```python
from build123d import *

# Parameters (mm, degrees)
F0_R     = 41.5925
F0_R_2   = 8.89
F1_DEPTH = 6.35
F2_R     = 41.5925
F2_R_2   = 33.9725
F3_DEPTH = 3.175
F4_R     = 41.5925
F4_R_2   = 33.9725
F4_R_3   = 0.762
F5_DEPTH = 2.54
F7_DEPTH = 6.985
F8_R     = 41.5925
F8_W     = 50.8
F8_H     = 50.8
F8_R_2   = 8.89
F8_R_3   = 8.382
F9_DEPTH = 12.7


with BuildPart() as f1:
    # F0 (on Top) → F1 (new body)
    with BuildSketch(Plane.XY):
        Circle(F0_R)
        Circle(F0_R_2, mode=Mode.SUBTRACT)
    extrude(amount=F1_DEPTH)

    # F2 (on face) → F3 (join)
    with BuildSketch(Plane.XY.offset(6.35)):
        Circle(F2_R)
        Circle(F2_R_2, mode=Mode.SUBTRACT)
    extrude(amount=F3_DEPTH)

    # F4 (on face) → F5 (join)
    with BuildSketch(Plane.XY.offset(9.525)):
        Circle(F4_R)
        Circle(F4_R_2, mode=Mode.SUBTRACT)
        Circle(F4_R_2)
        with Locations((-18.7126454725, -21.5955440872)):
            Circle(F4_R_3, mode=Mode.SUBTRACT)
        with Locations((-14.2875, -24.7466759131)):
            Circle(F4_R_3, mode=Mode.SUBTRACT)
        with Locations((-9.3459670518, -27.0033983948)):
            Circle(F4_R_3, mode=Mode.SUBTRACT)
        with Locations((-4.0666465037, -28.2841477017)):
            Circle(F4_R_3, mode=Mode.SUBTRACT)
        with Locations((-6.5563218998, -21.8996402515)):
            Circle(F4_R_3, mode=Mode.SUBTRACT)
        with Locations((-1.3291907889, -22.8213244981)):
            Circle(F4_R_3, mode=Mode.SUBTRACT)
        with Locations((-22.4614671823, -17.6638930313)):
            Circle(F4_R_3, mode=Mode.SUBTRACT)
        with Locations((-25.3984729453, -13.0938228584)):
            Circle(F4_R_3, mode=Mode.SUBTRACT)
        with Locations((-27.417511721, -8.0505078117)):
            Circle(F4_R_3, mode=Mode.SUBTRACT)
        with Locations((-21.4813733112, -7.8185804764)):
            Circle(F4_R_3, mode=Mode.SUBTRACT)
        with Locations((-28.4456101875, -2.7162264374)):
            Circle(F4_R_3, mode=Mode.SUBTRACT)
        with Locations((-22.705428858, -2.6538840169)):
            Circle(F4_R_3, mode=Mode.SUBTRACT)
        with Locations((-15.6874838417, -16.6277614464)):
            Circle(F4_R_3, mode=Mode.SUBTRACT)
        with Locations((-11.43, -19.7973407305)):
            Circle(F4_R_3, mode=Mode.SUBTRACT)
        with Locations((-19.0992513689, -12.5617752387)):
            Circle(F4_R_3, mode=Mode.SUBTRACT)
        with Locations((-5.2980963686, -16.3058639719)):
            Circle(F4_R_3, mode=Mode.SUBTRACT)
        with Locations((-10.0775781506, -13.8705963686)):
            Circle(F4_R_3, mode=Mode.SUBTRACT)
        with Locations((-4.0531338589, -10.6872356539)):
            Circle(F4_R_3, mode=Mode.SUBTRACT)
        with Locations((-16.3058639719, -5.2980963686)):
            Circle(F4_R_3, mode=Mode.SUBTRACT)
        with Locations((-13.8705963686, -10.0775781506)):
            Circle(F4_R_3, mode=Mode.SUBTRACT)
        with Locations((-11.0978649732, -2.7353780428)):
            Circle(F4_R_3, mode=Mode.SUBTRACT)
        with Locations((-8.5554778516, -7.5794919837)):
            Circle(F4_R_3, mode=Mode.SUBTRACT)
        with Locations((-2.8575, -4.9493351826)):
            Circle(F4_R_3, mode=Mode.SUBTRACT)
        with Locations((1.3596532447, -28.5426342172)):
            Circle(F4_R_3, mode=Mode.SUBTRACT)
        with Locations((6.7368115822, -27.7695155648)):
            Circle(F4_R_3, mode=Mode.SUBTRACT)
        with Locations((3.9695973415, -22.5127052339)):
            Circle(F4_R_3, mode=Mode.SUBTRACT)
        with Locations((9.0543834517, -20.9904202033)):
            Circle(F4_R_3, mode=Mode.SUBTRACT)
        with Locations((11.8704839965, -25.9927342673)):
            Circle(F4_R_3, mode=Mode.SUBTRACT)
        with Locations((16.575126191, -23.2765078298)):
            Circle(F4_R_3, mode=Mode.SUBTRACT)
        with Locations((0, -17.145)):
            Circle(F4_R_3, mode=Mode.SUBTRACT)
        with Locations((5.2980963686, -16.3058639719)):
            Circle(F4_R_3, mode=Mode.SUBTRACT)
        with Locations((1.3777342553, -11.3466624309)):
            Circle(F4_R_3, mode=Mode.SUBTRACT)
        with Locations((10.0775781506, -13.8705963686)):
            Circle(F4_R_3, mode=Mode.SUBTRACT)
        with Locations((13.6510454063, -18.3365361864)):
            Circle(F4_R_3, mode=Mode.SUBTRACT)
        with Locations((20.6807001389, -19.7190077531)):
            Circle(F4_R_3, mode=Mode.SUBTRACT)
        with Locations((17.5117759697, -14.6941247574)):
            Circle(F4_R_3, mode=Mode.SUBTRACT)
        with Locations((6.4929800551, -9.4067055872)):
            Circle(F4_R_3, mode=Mode.SUBTRACT)
        with Locations((10.1207623732, -5.3117858565)):
            Circle(F4_R_3, mode=Mode.SUBTRACT)
        with Locations((2.8575, -4.9493351826)):
            Circle(F4_R_3, mode=Mode.SUBTRACT)
        with Locations((13.8705963686, -10.0775781506)):
            Circle(F4_R_3, mode=Mode.SUBTRACT)
        with Locations((20.4284421578, -10.2595492594)):
            Circle(F4_R_3, mode=Mode.SUBTRACT)
        with Locations((16.3058639719, -5.2980963686)):
            Circle(F4_R_3, mode=Mode.SUBTRACT)
        with Locations((24.0388197007, -15.4488113588)):
            Circle(F4_R_3, mode=Mode.SUBTRACT)
        with Locations((26.5281136859, -10.6202546705)):
            Circle(F4_R_3, mode=Mode.SUBTRACT)
        with Locations((22.2438057415, -5.2718788052)):
            Circle(F4_R_3, mode=Mode.SUBTRACT)
        with Locations((28.0586125243, -5.4078543076)):
            Circle(F4_R_3, mode=Mode.SUBTRACT)
        with Locations((-28.4456101875, 2.7162264374)):
            Circle(F4_R_3, mode=Mode.SUBTRACT)
        with Locations((-22.705428858, 2.6538840169)):
            Circle(F4_R_3, mode=Mode.SUBTRACT)
        with Locations((-27.417511721, 8.0505078117)):
            Circle(F4_R_3, mode=Mode.SUBTRACT)
        with Locations((-21.4813733112, 7.8185804764)):
            Circle(F4_R_3, mode=Mode.SUBTRACT)
        with Locations((-25.3984729453, 13.0938228584)):
            Circle(F4_R_3, mode=Mode.SUBTRACT)
        with Locations((-22.4614671823, 17.6638930313)):
            Circle(F4_R_3, mode=Mode.SUBTRACT)
        with Locations((-17.145, 0)):
            Circle(F4_R_3, mode=Mode.SUBTRACT)
        with Locations((-11.0978649732, 2.7353780428)):
            Circle(F4_R_3, mode=Mode.SUBTRACT)
        with Locations((-16.3058639719, 5.2980963686)):
            Circle(F4_R_3, mode=Mode.SUBTRACT)
        with Locations((-13.8705963686, 10.0775781506)):
            Circle(F4_R_3, mode=Mode.SUBTRACT)
        with Locations((-5.715, 0)):
            Circle(F4_R_3, mode=Mode.SUBTRACT)
        with Locations((-2.8575, 4.9493351826)):
            Circle(F4_R_3, mode=Mode.SUBTRACT)
        with Locations((-8.5554778516, 7.5794919837)):
            Circle(F4_R_3, mode=Mode.SUBTRACT)
        with Locations((-19.0992513689, 12.5617752387)):
            Circle(F4_R_3, mode=Mode.SUBTRACT)
        with Locations((-15.6874838417, 16.6277614464)):
            Circle(F4_R_3, mode=Mode.SUBTRACT)
        with Locations((-11.43, 19.7973407305)):
            Circle(F4_R_3, mode=Mode.SUBTRACT)
        with Locations((-10.0775781506, 13.8705963686)):
            Circle(F4_R_3, mode=Mode.SUBTRACT)
        with Locations((-4.0531338589, 10.6872356539)):
            Circle(F4_R_3, mode=Mode.SUBTRACT)
        with Locations((-5.2980963686, 16.3058639719)):
            Circle(F4_R_3, mode=Mode.SUBTRACT)
        with Locations((-18.7126454725, 21.5955440872)):
            Circle(F4_R_3, mode=Mode.SUBTRACT)
        with Locations((-14.2875, 24.7466759131)):
            Circle(F4_R_3, mode=Mode.SUBTRACT)
        with Locations((-6.5563218998, 21.8996402515)):
            Circle(F4_R_3, mode=Mode.SUBTRACT)
        with Locations((-1.3291907889, 22.8213244981)):
            Circle(F4_R_3, mode=Mode.SUBTRACT)
        with Locations((-9.3459670518, 27.0033983948)):
            Circle(F4_R_3, mode=Mode.SUBTRACT)
        with Locations((-4.0666465037, 28.2841477017)):
            Circle(F4_R_3, mode=Mode.SUBTRACT)
        Circle(F4_R_3, mode=Mode.SUBTRACT)
        with Locations((2.8575, 4.9493351826)):
            Circle(F4_R_3, mode=Mode.SUBTRACT)
        with Locations((5.715, 0)):
            Circle(F4_R_3, mode=Mode.SUBTRACT)
        with Locations((10.1207623732, 5.3117858565)):
            Circle(F4_R_3, mode=Mode.SUBTRACT)
        with Locations((6.4929800551, 9.4067055872)):
            Circle(F4_R_3, mode=Mode.SUBTRACT)
        with Locations((11.43, 0)):
            Circle(F4_R_3, mode=Mode.SUBTRACT)
        with Locations((17.145, 0)):
            Circle(F4_R_3, mode=Mode.SUBTRACT)
        with Locations((13.8705963686, 10.0775781506)):
            Circle(F4_R_3, mode=Mode.SUBTRACT)
        with Locations((16.3058639719, 5.2980963686)):
            Circle(F4_R_3, mode=Mode.SUBTRACT)
        with Locations((20.4284421578, 10.2595492594)):
            Circle(F4_R_3, mode=Mode.SUBTRACT)
        with Locations((1.3777342553, 11.3466624309)):
            Circle(F4_R_3, mode=Mode.SUBTRACT)
        with Locations((10.0775781506, 13.8705963686)):
            Circle(F4_R_3, mode=Mode.SUBTRACT)
        with Locations((0, 17.145)):
            Circle(F4_R_3, mode=Mode.SUBTRACT)
        with Locations((5.2980963686, 16.3058639719)):
            Circle(F4_R_3, mode=Mode.SUBTRACT)
        with Locations((17.5117759697, 14.6941247574)):
            Circle(F4_R_3, mode=Mode.SUBTRACT)
        with Locations((13.6510454063, 18.3365361864)):
            Circle(F4_R_3, mode=Mode.SUBTRACT)
        with Locations((20.6807001389, 19.7190077531)):
            Circle(F4_R_3, mode=Mode.SUBTRACT)
        with Locations((22.86, 0)):
            Circle(F4_R_3, mode=Mode.SUBTRACT)
        with Locations((28.575, 0)):
            Circle(F4_R_3, mode=Mode.SUBTRACT)
        with Locations((22.2438057415, 5.2718788052)):
            Circle(F4_R_3, mode=Mode.SUBTRACT)
        with Locations((28.0586125243, 5.4078543076)):
            Circle(F4_R_3, mode=Mode.SUBTRACT)
        with Locations((24.0388197007, 15.4488113588)):
            Circle(F4_R_3, mode=Mode.SUBTRACT)
        with Locations((26.5281136859, 10.6202546705)):
            Circle(F4_R_3, mode=Mode.SUBTRACT)
        with Locations((3.9695973415, 22.5127052339)):
            Circle(F4_R_3, mode=Mode.SUBTRACT)
        with Locations((9.0543834517, 20.9904202033)):
            Circle(F4_R_3, mode=Mode.SUBTRACT)
        with Locations((1.3596532447, 28.5426342172)):
            Circle(F4_R_3, mode=Mode.SUBTRACT)
        with Locations((6.7368115822, 27.7695155648)):
            Circle(F4_R_3, mode=Mode.SUBTRACT)
        with Locations((11.8704839965, 25.9927342673)):
            Circle(F4_R_3, mode=Mode.SUBTRACT)
        with Locations((16.575126191, 23.2765078298)):
            Circle(F4_R_3, mode=Mode.SUBTRACT)
    extrude(amount=F5_DEPTH)

    # F6 (on face) → F7 (join)
    with BuildSketch(Plane.XY.offset(12.065)):
        with BuildLine():
            ThreePointArc((18.8740600105, -37.0635388889), (35.4609320044, -21.7361072327), (41.5925, 0))
            ThreePointArc((41.5925, 0), (-29.4103387965, 29.4103387965), (0, -41.5925))
            Line((0, -41.5925), (0, -38.1))
            ThreePointArc((0, -38.1), (-26.9407683632, 26.9407683632), (38.1, 0))
            ThreePointArc((38.1, 0), (32.4832964926, -19.9109379231), (17.2892152768, -33.9513333333))
            Line((17.2892152768, -33.9513333333), (18.8740600105, -37.0635388889))
        make_face()
    extrude(amount=F7_DEPTH)

    # F8 (on face) → F9 (join)
    with BuildSketch(Plane(origin=(0, 0, 0), x_dir=(1, 0, 0), z_dir=(0, 0, -1))):
        Circle(F8_R)
        Rectangle(F8_W, F8_H, mode=Mode.SUBTRACT)
        Rectangle(F8_W, F8_H)
        Circle(F8_R_2, mode=Mode.SUBTRACT)
        Circle(F8_R_2)
        Circle(F8_R_3, mode=Mode.SUBTRACT)
    extrude(amount=F9_DEPTH)


solid = f1.part
```
Model file for the job. Use its own axes, mm. A direction names the side the tool comes from. Give positions to 0.01 mm unless a question says otherwise; leave off trailing zeros. Order: outer loops, then holes, each group sorted by start corner. A loop starts at its lowest first (then second) coordinate and runs counter-clockwise, first axis right, second up.
1) 3-axis set-ups, long thin cutter, end or side, ignore diameter. For faces 1 (the cylindrical face through (8, -2.5, -6.3)), 2 (the flat face through (7, 0, 9.525)), 3 (the flat face through (-1, 9, -12.7)): which of +Z, -Z, +X, -X, +Y, -Y reach the whole face in a straight line?
2) Mould opens along Y. For faces 4 (the cylindrical face through (38.95, -14.59, 3.4)), 5 (the flat face through (0, -40, 16)), 6 (the flat face through (-1, -1, 12.065)), 7 (the flat face through (18.071, -35.486, 15.509)) say: +Y half, -Y half, draft (parallel to the pull), parting line (faces both ways), or undercut.
3) Pin check, flat tips, straight feed: pin 1 (5 mm diameter, centred on x = -7.5, z = 4, fed in from -Y); pin 2 (2 mm diameter, centred on x = -15.69, y = 16.63, fed in from +Z) (3 decimals); pin 3 (1.2 mm diameter, centred on x = 9.05, y = 20.99, fed in from +Z). Stop position of each tip, or through.
4) Saw through at B-B, the plane y = 35. Write the cut outline in (x, z) (3 decimals), then the cut area to 3 significant figures.
5) Saw through at A-A, the plane z = 14.5. Write the cut outline in (x, y) (1 decimal), then the cut area to 3 significant figures.
6) Wall check: probe 1 along Z at (x, y) = (-30.5, 14) (3 decimals); probe 2 along Y at (x, z) = (0.5, 8.5); probe 3 along Y at (x, z) = (-1, 2). Give the ranges that are in metal, low to high.
Computed:
1. face 1: -Z
1. face 2: none
1. face 3: -Z, +X, -X, +Y, -Y
2. face 4: parting line
2. face 5: draft
2. face 6: undercut
2. face 7: -Y half
3. pin 1: stops at y = -41.29
3. pin 2: stops at z = 12.065
3. pin 3: stops at z = 6.35
4. outline: (-22.471, -12.7) - (22.471, -12.7) - (22.471, 19.05) - (15.054, 19.05) - (15.054, 12.065) - (-15.054, 12.065) - (-15.054, 19.05) - (-22.471, 19.05) - close
4. area: 1,220 mm2
5. outline: (0, -41.6) - (0, -38.1) arc R38.1 cw (long way) to (17.3, -34) - (18.9, -37.1) arc R41.6 ccw (long way) to start
5. area: 809 mm2
6. probe 1: z = -12.7 to 6.35, 9.525 to 12.065
6. probe 2: y = -41.59 to -33.97, 33.97 to 41.59
6. probe 3: y = -41.58 to -8.83, 8.83 to 41.58
